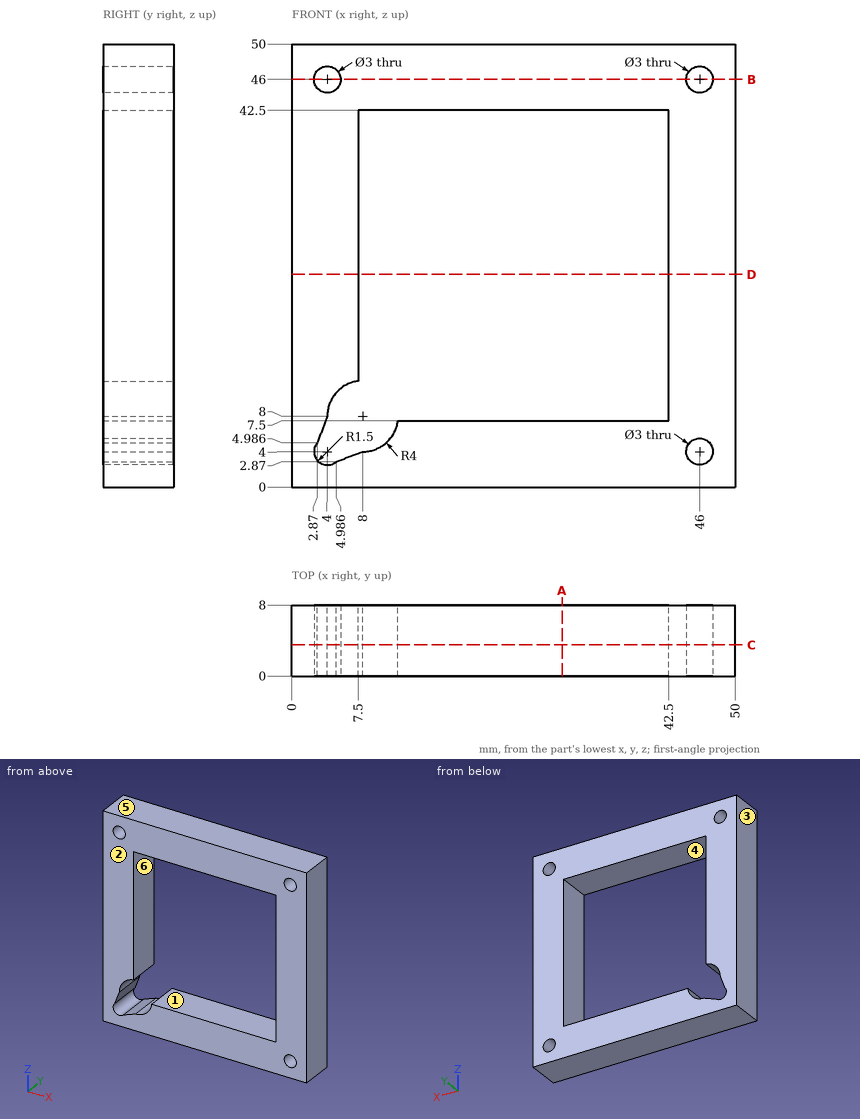
Job drawing, mm, ordinate dimensions from the low corner. One solid piece. A direction names the side the tool comes from. Coordinates: 2 decimals unless noted, no trailing zeros. Loops run counter-clockwise (first coordinate to the right, second up) from the corner with the lowest first, then second, coordinate; pieces in that order, holes last. Notation, with made-up numbers: (83.25, 53) - (114.25, 53) arc R25 ccw to (114.25, 87) - close; hole circle Ø7 at (44, 18). An arc over 180 degrees is marked (long way). Answer as a JSON object with one key per item and string values. Group by question number.
(1) Probe line 1 along X through (y, z) = (6, 46); line 2 along Z through (x, y) = (38.5, 7.5). List the from-to ranges inside material, lowest first.
(2) Cut at A-A (x = 30.5). Give the cut face in (y, z).
(3) Two-plate mould, pull along Z, no slides. Class the marked faces 3, 4, 5 and 6: released by +Z, released by -Z, zero draft, split by the parting line, or undercut.
(4) Tool access for the marked faces 1 and 2: list every direction of +Z, -Z, +X, -X, +Y, -Y with a clear straight run to the whole face (end or side of a thin tool).
(5) Cut at C-C (y = 3.5). Give the cut face in (x, z).
(6) Cut at B-B (z = 46). Give the cut face in (x, y).
(7) Cut at D-D (z = 24). Give the cut face in (x, y).
Geometry says:
{
 "1": {"line 1": "x = 0 to 2.5, 5.5 to 44.5, 47.5 to 50", "line 2": "z = 0 to 7.5, 42.5 to 50"},
 "2": {"outline": "(0, 0) - (8, 0) - (8, 7.5) - (0, 7.5) - close; (0, 42.5) - (8, 42.5) - (8, 50) - (0, 50) - close"},
 "3": {"face 3": "zero draft", "face 4": "undercut", "face 5": "released by +Z", "face 6": "undercut"},
 "4": {"face 1": "+Y, -Y", "face 2": "+Z, -Z, +X, -X, -Y"},
 "5": {"outline": "(0, 0) - (50, 0) - (50, 50) - (0, 50) - close; hole circle Ø3 at (4, 46); hole (2.87, 4.99) arc R1.5 ccw to (4.99, 2.87) - (8, 4) arc R4 ccw to (11.97, 7.5) - (42.5, 7.5) - (42.5, 42.5) - (7.5, 42.5) - (7.5, 11.97) arc R4 ccw to (4, 8) - close; hole circle Ø3 at (46, 4); hole circle Ø3 at (46, 46)"},
 "6": {"outline": "(0, 0) - (2.5, 0) - (2.5, 8) - (0, 8) - close; (5.5, 0) - (44.5, 0) - (44.5, 8) - (5.5, 8) - close; (47.5, 0) - (50, 0) - (50, 8) - (47.5, 8) - close"},
 "7": {"outline": "(0, 0) - (7.5, 0) - (7.5, 8) - (0, 8) - close; (42.5, 0) - (50, 0) - (50, 8) - (42.5, 8) - close"}
}
